```python
from build123d import *

# Parameters (mm, degrees)
SKETCH2_R           = 25
BOSS_EXTRUDE1_DEPTH = 14.6
SKETCH3_R           = 33.5
SKETCH3_R_2         = 25
BOSS_EXTRUDE2_DEPTH = 40
SKETCH6_W           = 14
SKETCH6_H           = 12
CUT_EXTRUDE1_DEPTH  = 64
CHAMFER1_SIZE       = 1.5


with BuildPart() as part:
    # Sketch2 → Boss-Extrude1 (new body)
    with BuildSketch(Plane.XY):
        with BuildLine():
            ThreePointArc((-18.974755856, 42.454209074), (-22.172929883, 45.798002784), (-25.900754962, 48.538913885))
            ThreePointArc((-25.900754962, 48.538913885), (-27.508522628, 47.646158833), (-29.085555016, 46.700168716))
            ThreePointArc((-29.085555016, 46.700168716), (-28.575768912, 42.101321947), (-27.279045628, 37.659725139))
            ThreePointArc((-27.279045628, 37.659725139), (-29.082617414, 29.082617413), (-37.659725139, 27.279045628))
            ThreePointArc((-37.659725139, 27.279045628), (-42.101321947, 28.575768912), (-46.700168717, 29.085555016))
            ThreePointArc((-46.700168717, 29.085555016), (-47.646158833, 27.508522628), (-48.538913885, 25.900754962))
            ThreePointArc((-48.538913885, 25.900754962), (-45.798002784, 22.172929883), (-42.454209074, 18.974755856))
            ThreePointArc((-42.454209074, 18.974755856), (-39.727594195, 10.644976782), (-46.253801484, 4.794483935))
            ThreePointArc((-46.253801484, 4.794483935), (-50.748698795, 3.696680837), (-54.986309977, 1.838745168))
            ThreePointArc((-54.986309977, 1.838745168), (-55.017045256, 0), (-54.986309977, -1.838745169))
            ThreePointArc((-54.986309977, -1.838745169), (-50.748698795, -3.696680837), (-46.253801484, -4.794483935))
            ThreePointArc((-46.253801484, -4.794483935), (-39.727594195, -10.644976782), (-42.454209074, -18.974755856))
            ThreePointArc((-42.454209074, -18.974755856), (-45.798002784, -22.172929883), (-48.538913885, -25.900754962))
            ThreePointArc((-48.538913885, -25.900754962), (-47.646158833, -27.508522628), (-46.700168717, -29.085555016))
            ThreePointArc((-46.700168717, -29.085555016), (-42.101321947, -28.575768912), (-37.659725139, -27.279045628))
            ThreePointArc((-37.659725139, -27.279045628), (-29.082617413, -29.082617414), (-27.279045628, -37.659725139))
            ThreePointArc((-27.279045628, -37.659725139), (-28.575768912, -42.101321947), (-29.085555016, -46.700168717))
            ThreePointArc((-29.085555016, -46.700168717), (-27.508522628, -47.646158833), (-25.900754962, -48.538913885))
            ThreePointArc((-25.900754962, -48.538913885), (-22.172929883, -45.798002784), (-18.974755856, -42.454209074))
            ThreePointArc((-18.974755856, -42.454209074), (-10.644976782, -39.727594195), (-4.794483935, -46.253801484))
            ThreePointArc((-4.794483935, -46.253801484), (-3.696680837, -50.748698795), (-1.838745168, -54.986309977))
            ThreePointArc((-1.838745168, -54.986309977), (0, -55.017045256), (1.838745168, -54.986309977))
            ThreePointArc((1.838745168, -54.986309977), (3.696680837, -50.748698795), (4.794483935, -46.253801484))
            ThreePointArc((4.794483935, -46.253801484), (10.644976782, -39.727594195), (18.974755856, -42.454209074))
            ThreePointArc((18.974755856, -42.454209074), (22.172929883, -45.798002784), (25.900754962, -48.538913885))
            ThreePointArc((25.900754962, -48.538913885), (27.508522628, -47.646158833), (29.085555016, -46.700168716))
            ThreePointArc((29.085555016, -46.700168716), (28.575768912, -42.101321947), (27.279045628, -37.659725139))
            ThreePointArc((27.279045628, -37.659725139), (29.082617413, -29.082617414), (37.659725139, -27.279045628))
            ThreePointArc((37.659725139, -27.279045628), (42.101321947, -28.575768912), (46.700168716, -29.085555016))
            ThreePointArc((46.700168716, -29.085555016), (47.646158833, -27.508522628), (48.538913885, -25.900754962))
            ThreePointArc((48.538913885, -25.900754962), (45.798002784, -22.172929883), (42.454209074, -18.974755856))
            ThreePointArc((42.454209074, -18.974755856), (39.727594195, -10.644976782), (46.253801483, -4.794483935))
            ThreePointArc((46.253801483, -4.794483935), (50.748698795, -3.696680837), (54.986309977, -1.838745168))
            ThreePointArc((54.986309977, -1.838745168), (55.017045256, 0), (54.986309977, 1.838745169))
            ThreePointArc((54.986309977, 1.838745169), (50.748698795, 3.696680837), (46.253801484, 4.794483935))
            ThreePointArc((46.253801484, 4.794483935), (39.727594195, 10.644976782), (42.454209074, 18.974755856))
            ThreePointArc((42.454209074, 18.974755856), (45.798002784, 22.172929883), (48.538913885, 25.900754962))
            ThreePointArc((48.538913885, 25.900754962), (47.646158833, 27.508522628), (46.700168717, 29.085555015))
            ThreePointArc((46.700168717, 29.085555015), (42.101321947, 28.575768912), (37.659725139, 27.279045628))
            ThreePointArc((37.659725139, 27.279045628), (29.082617413, 29.082617413), (27.279045628, 37.659725139))
            ThreePointArc((27.279045628, 37.659725139), (28.575768912, 42.101321947), (29.085555016, 46.700168717))
            ThreePointArc((29.085555016, 46.700168717), (27.508522628, 47.646158833), (25.900754962, 48.538913885))
            ThreePointArc((25.900754962, 48.538913885), (22.172929883, 45.798002784), (18.974755856, 42.454209074))
            ThreePointArc((18.974755856, 42.454209074), (10.644976782, 39.727594195), (4.794483935, 46.253801483))
            ThreePointArc((4.794483935, 46.253801483), (3.696680837, 50.748698795), (1.838745168, 54.986309977))
            ThreePointArc((1.838745168, 54.986309977), (0, 55.017045256), (-1.838745168, 54.986309977))
            ThreePointArc((-1.838745168, 54.986309977), (-3.696680837, 50.748698795), (-4.794483935, 46.253801483))
            ThreePointArc((-4.794483935, 46.253801483), (-10.644976782, 39.727594195), (-18.974755856, 42.454209074))
        make_face()
        Circle(SKETCH2_R, mode=Mode.SUBTRACT)
    extrude(amount=BOSS_EXTRUDE1_DEPTH)

    # Sketch3 → Boss-Extrude2 (add)
    with BuildSketch(Plane(origin=(0, 0, 0), x_dir=(-1, 0, 0), z_dir=(0, 0, -1))):
        Circle(SKETCH3_R)
        Circle(SKETCH3_R_2, mode=Mode.SUBTRACT)
    extrude(amount=-BOSS_EXTRUDE2_DEPTH)

    # Sketch6 → Cut-Extrude1 (cut)
    with BuildSketch(Plane.XY.offset(40)):
        with Locations((0, 23.3)):
            Rectangle(SKETCH6_W, SKETCH6_H)
    extrude(amount=-CUT_EXTRUDE1_DEPTH, mode=Mode.SUBTRACT)

    # Chamfer1
    chamfer1_edges = [part.edges().sort_by_distance(p)[0] for p in [
        (33.5, 0, 14.6),
        (33.5, 0, 40),
        (15, -20, 40),
    ]]
    chamfer(chamfer1_edges, length=CHAMFER1_SIZE)


solid = part.part
```
CAD build for the part. Positions are in the model's coordinates, mm. A direction names the side the tool comes from. Coordinates: 2 decimals unless noted, no trailing zeros. Order: outer loops, then holes, each group sorted by start corner. A loop starts at its lowest first (then second) coordinate and runs counter-clockwise, first axis right, second up. Notation, with made-up numbers: M 79,-5 L 101,-5 A22 cw 101,19 Z; hole C 79.5,36 d6. An arc over 180 degrees is marked long. Answer as CSV lines item,"result".
1) Cut at A-A (x = 0). List the corners of the cut face in (y, z).
Verdict:
outline,"M -55.02,0 L -25,0 L -25,38.5 L -26.5,40 L -32,40 L -33.5,38.5 L -33.5,16.1 L -35,14.6 L -55.02,14.6 Z; M 29.3,0 L 55.02,0 L 55.02,14.6 L 35,14.6 L 33.5,16.1 L 33.5,38.5 L 32,40 L 29.3,40 Z"
2) Cut at B-B (z = 22.5). List the corners of the cut face in (x, y).
Verdict:
outline,"C 0,0 d67; hole M -7,24 A25 ccw long 7,24 L 7,29.3 L -7,29.3 Z"
3) Flat gauge pins, fed straight in: P1, Ø4, axis at x = 8, z = 25, coming from the -Y side; P2, Ø3, axis at y = 10, z = 23.5, coming from the +X side; P3, Ø10, axis at x = 21, z = 26, coming from the -Y side. Where does each tip first touch, or does it go through?
Verdict:
P1,"y = -32.96"
P2,"x = 32.4"
P3,"y = -29.43"
4) Drill centre lines: L1, parallel to X at y = 0, z = 11; L2, parallel to X at y = -1, z = 19; L3, parallel to Y at x = 0, z = 10. Where is each one in solid material? Low to high. Write a range as from..to.
Verdict:
L1,"-55.02..-25, 25..55.02"
L2,"-33.49..-24.98, 24.98..33.49"
L3,"-55.02..-25, 29.3..55.02"
5) Mould opens along Y. For faces 4 (the cylindrical face through (-22.124, 45.755, 7.198)), 5 (the cylindrical face through (-27.531, -47.633, 7.198)), 6 (the cylindrical face through (-50.687, 3.717, 7.198)) say: released by +Y, released by -Y, zero draft, split by the parting line, or undercut.
Verdict:
face 4,"released by +Y"
face 5,"released by -Y"
face 6,"undercut"
6) 3-axis set-ups, long thin cutter, end or side, ignore diameter. For faces 1 (the cylindrical face through (-28.563, -42.038, 7.198)), 2 (the flat face through (-7, 27, 20)), 3 (the flat face through (-29, 21, 14.6)): which of +Z, -Z, +X, -X, +Y, -Y reach the whole face in a straight line?
Verdict:
face 1,"+Z, -Z, -X"
face 2,"+Z, -Z"
face 3,"+Z"
